from build123d import *

# Parameters (mm, degrees)
F1_DEPTH = 11.1125


# Not quite as in the source:
# - a length typed as a fraction of an inch, garbled in the dataset ("3 / 203.2 mm" for 3/8 in), is restored


with BuildPart() as f1:
    # F0 (on Top) → F1 (new body)
    with BuildSketch(Plane.XY):
        with BuildLine():
            ThreePointArc((-0.1411418198, 20.1985444874), (-5.0054503986, 18.2564119782), (-9.2097157612, 15.1327075437))
            ThreePointArc((-9.2097157612, 15.1327075437), (-10.6205392688, 11.8246856933), (-10.2093555033, 8.2519613206))
            Line((-10.2093555033, 8.2519613206), (-12.369341217, 7.1464567445))
            Line((-12.369341217, 7.1464567445), (-12.369341217, 4.6386048198))
            Line((-12.369341217, 4.6386048198), (-12.369341217, 4.5682978211))
            ThreePointArc((-12.369341217, 4.5682978211), (-15.5930977879, 3.1185654947), (-17.7027139134, 0.2823972963))
            ThreePointArc((-17.7027139134, 0.2823972963), (-21.0452825194, -1.0603738309), (-23.1384971151, -3.9919692741))
            ThreePointArc((-23.1384971151, -3.9919692741), (-23.9954710425, -8.6613028545), (-23.5336683691, -13.3861117065))
            ThreePointArc((-23.5336683691, -13.3861117065), (-19.6562098094, -16.4130421994), (-15.0192606046, -18.054899429))
            ThreePointArc((-15.0192606046, -18.054899429), (-11.4338171794, -17.7079201351), (-8.5996589687, -15.484556372))
            ThreePointArc((-8.5996589687, -15.484556372), (-5.0294162563, -15.0523544446), (-2.1409380715, -12.9098966718))
            Line((-2.1409380715, -12.9098966718), (0, -14.2561570176))
            Line((0, -14.2561570176), (1.9696742658, -12.9098966718))
            ThreePointArc((1.9696742658, -12.9098966718), (4.9392756736, -15.0084468105), (8.560301624, -15.3410370587))
            ThreePointArc((8.560301624, -15.3410370587), (11.3944598347, -17.5644008218), (14.9799032599, -17.9113801157))
            ThreePointArc((14.9799032599, -17.9113801157), (19.5156578324, -16.3470620723), (23.423301056, -13.563092798))
            ThreePointArc((23.423301056, -13.563092798), (23.8861103651, -8.6849198531), (23.0991397704, -3.8484499608))
            ThreePointArc((23.0991397704, -3.8484499608), (21.0059251747, -0.9168545176), (17.6633565687, 0.4259166096))
            ThreePointArc((17.6633565687, 0.4259166096), (15.4847616458, 3.3168082822), (12.1560195839, 4.739132713))
            Line((12.1560195839, 4.739132713), (12.1560195839, 7.1464567445))
            Line((12.1560195839, 7.1464567445), (9.9960338703, 8.2519613206))
            ThreePointArc((9.9960338703, 8.2519613206), (10.4072176357, 11.8246856933), (8.9963941282, 15.1327075437))
            ThreePointArc((8.9963941282, 15.1327075437), (4.7823081966, 18.3053860292), (-0.1411418198, 20.1985444874))
        make_face()
    extrude(amount=F1_DEPTH)


solid = f1.part
The model under review builds one solid part; all positions refer to its coordinate system, in mm. A direction names the side the tool comes from. Coordinates: 2 decimals unless noted, no trailing zeros. Loops run counter-clockwise (first coordinate to the right, second up) from the corner with the lowest first, then second, coordinate; pieces in that order, holes last. Notation, with made-up numbers: (-31, 7.25) -> (11, 7.25) arc R9 ccw to (11, 15.25) -> close; hole circle Ø4 at (75, -37). An arc over 180 degrees is marked (long way). Use a Markdown table: item, result. Add a question column.
1. Clearance check with flat-ended pins moving along their axes: pin 1 Ø1 at (y, z) = (-14, 5) entering from -X; pin 2 Ø5 at (y, z) = (-12.5, 9) entering from +X; pin 3 Ø4 at (y, z) = (7.5, 8.5) entering from +X. State where each tip first meets the part, or that it passes through.
2. Draft analysis for pull direction X (two halves, no side actions). For faces 1 (the face through (0.971, -13.592, 5.478)), 2 (the face through (19.456, -16.378, 5.478)), 3 (the face through (-12.369, 6, 5)), state which applies: pulls with the +X half, pulls with the -X half, needs draft (parallel to the pull), parting line crosses it, or undercut.
3. Add section A-A on z = 7.75. Write out the cut boundary in (x, y).
4. Add section B-B on y = -0.5. Write out the cut boundary in (x, z).
5. Machinability: for faces 4 (the face through (-1.09, -13.57, 5.48)), 5 (the face through (11.09, 7.69, 5.48)), 6 (the face through (12.156, 6, 5)), which of the approach directions +Z, -Z, +X, -X, +Y, -Y give a long, thin tool a straight path to every point of the face, cutting with its end or side? Answer none if there is none.
6. To check wall thickness, follow line 1 (Y direction, x = -17, z = 6); line 2 (X direction, y = 14, z = 8.5); line 3 (Y direction, x = -4, z = 10.5). State the ranges of each line that lie inside material, in increasing order.
7. Add section C-C on x = -3. Write out the cut boundary in (y, z).
Returned:
| question | item | result |
|---|---|---|
| 1 | pin 1 | stops at x = -23.43 |
| 1 | pin 2 | stops at x = 23.88 |
| 1 | pin 3 | stops at x = 12.16 |
| 2 | face 1 | undercut |
| 2 | face 2 | pulls with the +X half |
| 2 | face 3 | pulls with the -X half |
| 3 | outline | (-23.53, -13.39) arc R15.32 ccw to (-15.02, -18.05) arc R6.42 ccw to (-8.6, -15.48) arc R7.02 ccw to (-2.14, -12.91) -> (0, -14.26) -> (1.97, -12.91) arc R7.02 ccw to (8.56, -15.34) arc R6.42 ccw to (14.98, -17.91) arc R16.78 ccw to (23.42, -13.56) arc R19.2 ccw to (23.1, -3.85) arc R6.42 ccw to (17.66, 0.43) arc R7.02 ccw to (12.16, 4.74) -> (12.16, 7.15) -> (10, 8.25) arc R7.02 ccw to (9, 15.13) arc R19.02 ccw to (-0.14, 20.2) arc R20.27 ccw to (-9.21, 15.13) arc R7.02 ccw to (-10.21, 8.25) -> (-12.37, 7.15) -> (-12.37, 4.57) arc R7.02 ccw to (-17.7, 0.28) arc R6.42 ccw to (-23.14, -3.99) arc R17.07 ccw to start |
| 4 | outline | (-20.2, 0) -> (20.41, 0) -> (20.41, 11.11) -> (-20.2, 11.11) -> close |
| 5 | face 4 | +Z, -Z, -Y |
| 5 | face 5 | +Z, -Z, +X |
| 5 | face 6 | +Z, -Z, +X, +Y |
| 6 | line 1 | y = -17.56 to 1.6 |
| 6 | line 2 | x = -9.93 to 9.72 |
| 6 | line 3 | y = -14.54 to 18.78 |
| 7 | outline | (-13.81, 0) -> (19.24, 0) -> (19.24, 11.11) -> (-13.81, 11.11) -> close |
